```python
from build123d import *

# Parameters (mm, degrees)
THICKEN1_T2   = 1
CHAMFER1_SIZE = 0.04


with BuildPart() as body_1:
    # Surface-Revolve1: a surface, the sketch's curves turned about an axis
    with BuildLine(Plane.XY, mode=Mode.PRIVATE) as surface_revolve1_1_path:
        Line((2, 0), (2, 27))
        ThreePointArc((2, 27), (1.414213562, 28.414213562), (0, 29))
    surface_revolve1_1 = Shell.revolve(surface_revolve1_1_path.wire(), 360, Axis((0, 0, 0), (0, 1, 0)))
    add(Solid.thicken(surface_revolve1_1, -THICKEN1_T2))

    # Sketch2 → Revolve1 (revolve)
    with BuildSketch(Plane.XY, mode=Mode.PRIVATE) as revolve1_sk:
        with BuildLine():
            Line((0, 29), (0, 27))
            Line((0, 27), (-2, 27))
            ThreePointArc((-2, 27), (-1.414213562, 28.414213562), (0, 29))
        make_face()
    revolve(revolve1_sk.sketch.rotate(Axis((0, 29, 0), (0, -1, 0)), 270), axis=Axis((0, 29, 0), (0, -1, 0)))

    # Chamfer1
    chamfer1_edges = [body_1.edges().sort_by_distance(p)[0] for p in [
        (-2, 0, 0),
    ]]
    chamfer(chamfer1_edges, length=CHAMFER1_SIZE)


solid = body_1.part
```
Model file for the job. Use its own axes, mm. Coordinates: 2 decimals unless noted, no trailing zeros. Loops run counter-clockwise (first coordinate to the right, second up) from the corner with the lowest first, then second, coordinate; pieces in that order, holes last. Notation, with made-up numbers: M 18.5,89 L 31.5,89 A22 cw 31.5,104 Z; hole C 32.25,-38.75 d10. An arc over 180 degrees is marked long. Use CSV: the item, a comma, the result in double quotes. Start each with the question number.
1. Band-saw the part on A-A, the plane z = 0. List the corners of the cut face in (x, y), then the cut area to 3 significant figures.
2. Flat gauge pin, fed straight in: pin 1 (1.6 mm diameter, centred on x = 0, z = 0, fed in from -Y). Where does the tip first touch, or does it go through?
3. Band-saw the part on B-B, the plane x = 0. List the corners of the cut face in (y, z), then the cut area to 3 significant figures.
4. Two-plate mould, pull along X, no slides. Class faces 1 (the cylindrical face through (0, 14, 1)), 2 (the cylindrical face through (0, 14, 2)), 3 (the flat face through (-1, 0, 1)): pulls with the +X half, pulls with the -X half, needs draft (parallel to the pull), parting line crosses it, or undercut.
5. Band-saw the part on C-C, the plane y = 5.5. List the corners of the cut face in (x, z).
6. Probe probe 1 along Z at (x, y) = (0, 18.75); probe 2 along X at (y, z) = (18.5, -0.9). List the from-to ranges inside material, lowest first. Write a range as [from, to].
Entries:
1,outline,"M -2,0.04 L -1.96,0 L -1,0 L -1,27 L 1,27 L 1,0 L 1.96,0 L 2,0.04 L 2,27 A2 ccw -2,27 Z"
1,area,"60.3 mm2"
2,pin 1,"stops at y = 27"
3,outline,"M 0,-1.96 L 0.04,-2 L 27,-2 A2 ccw 27,2 L 0.04,2 L 0,1.96 L 0,1 L 27,1 L 27,-1 L 0,-1 Z"
3,area,"60.3 mm2"
4,face 1,"undercut"
4,face 2,"parting line crosses it"
4,face 3,"needs draft"
5,outline,"C 0,0 d4; hole C 0,0 d2"
6,probe 1,"z = [-2, -1], [1, 2]"
6,probe 2,"x = [-1.79, -0.44], [0.44, 1.79]"
